Here's how the part is built. I have some questions about the finished solid (model axes, mm). A direction names the side the tool comes from. Round coordinates to 2 decimals unless told otherwise and drop trailing zeros. Write each loop counter-clockwise with the first axis right and the second up, starting at its lowest first coordinate (ties: lowest second). Pieces come first, ordered by that corner, then holes. Notation, with made-up numbers: (-14.5, 38) -> (30.5, 38) arc R15 cw to (30.5, 59) -> close; hole circle Ø8 at (-3.75, 35). An arc over 180 degrees is marked (long way). Answer as CSV lines item,"result".
```python
from build123d import *

# Parameters (mm, degrees)
F0_W     = 150
F0_H     = 50
F1_DEPTH = 20
F2_T     = -2.54
F3_DEPTH = 5
F4_R     = 16.256


with BuildPart() as f1:
    # F0 (on Top) → F1 (new body)
    with BuildSketch(Plane.XY):
        with Locations((1.6509965062, -8.4789711357)):
            Rectangle(F0_W, F0_H)
    extrude(amount=F1_DEPTH)

    # F2
    f2_openings = [f1.faces().sort_by_distance(p)[0] for p in [
        (1.650997, -33.478971, 10),
    ]]
    offset(amount=F2_T, openings=f2_openings)

    # F3 (add): a face of the model
    f3_faces = [f1.faces().sort_by_distance(p)[0] for p in [
        (1.6509965062, 16.5210288643, 10),
    ]]
    extrude(f3_faces, amount=F3_DEPTH)

    # F4
    f4_edges = [f1.edges().sort_by_distance(p)[0] for p in [
        (1.650997, 21.521029, 20),
    ]]
    fillet(f4_edges, radius=F4_R)


solid = f1.part
```
1. Suppose I cut it at C-C on z = 7.5. Please give me the cut outline in (x, y), and give its area (3 significant figures).
Numbers:
outline,"(-73.35, -33.48) -> (-70.81, -33.48) -> (-70.81, 13.98) -> (74.11, 13.98) -> (74.11, -33.48) -> (76.65, -33.48) -> (76.65, 21.08) -> (-73.35, 21.08) -> close"
area,"1,310 mm^2"
2. On a 3-axis mill with a long thin cutter (end or side, diameter ignored), from which of +Z, -Z, +X, -X, +Y, -Y can I reach the whole of each face in a straight line? I mean faces 5 (the face through (1, 13.981, 10)), 6 (the face through (76.651, -6, 10)). Say none if no direction works.
Numbers:
face 5,"-Y"
face 6,"+Z, -Z, +X, +Y, -Y"
3. If we mould it in two halves opening along Z, with no side actions, what happens to faces 1 (the face through (74.111, -10, 10)), 2 (the face through (2.701, 16.633, 15.364)), 3 (the face through (-70.809, -10, 10)), 4 (the face through (-10, -33.479, 18))? For each: released by +Z, released by -Z, zero draft, split by the parting line, or undercut.
Numbers:
face 1,"undercut"
face 2,"released by +Z"
face 3,"undercut"
face 4,"zero draft"
4. If I drill on line 1 (Z direction, x = 6.5, y = -27); line 2 (X direction, y = -6.5, z = 10); line 3 (Y direction, x = -45.5, z = 3), over which ranges is the centre line in solid material (lowest first)?
Numbers:
line 1,"z = 0 to 2.54, 17.46 to 20"
line 2,"x = -73.35 to -70.81, 74.11 to 76.65"
line 3,"y = 13.98 to 21.52"
5. Suppose I cut it at D-D on y = 12. Please give me the cut outline in (x, z), and give its area (3 significant figures).
Numbers:
outline,"(-73.35, 0) -> (76.65, 0) -> (76.65, 18.54) -> (-73.35, 18.54) -> close; hole (-70.81, 2.54) -> (74.11, 2.54) -> (74.11, 17.46) -> (-70.81, 17.46) -> close"
area,"619 mm^2"
6. Suppose I cut it at A-A on x = -51. Please give me the cut outline in (y, z).
Numbers:
outline,"(-33.48, 0) -> (21.52, 0) -> (21.52, 3.74) arc R16.26 ccw to (5.27, 20) -> (-33.48, 20) -> (-33.48, 17.46) -> (13.98, 17.46) -> (13.98, 2.54) -> (-33.48, 2.54) -> close"
7. Suppose I cut it at B-B on y = -26.5. Please give me the cut outline in (x, z), and give its area (3 significant figures).
Numbers:
outline,"(-73.35, 0) -> (76.65, 0) -> (76.65, 20) -> (-73.35, 20) -> close; hole (-70.81, 2.54) -> (74.11, 2.54) -> (74.11, 17.46) -> (-70.81, 17.46) -> close"
area,"838 mm^2"
